```python
from build123d import *

# Parameters (mm, degrees)
F0_W           = 1549.4
F0_H           = 254
F1_DEPTH       = 12.7
F3_D           = 6.6
F3_CBORE_D     = 11.25
F3_CBORE_DEPTH = 6
F4_W           = 7.62
F4_H           = 5.5372
F6_DEPTH       = 12.7
F8_D           = 26.59126
F10_D          = 9.5758
F12_DEPTH      = 25.4
F13_R          = 9.525


with BuildPart() as f1:
    # F0 (on Front) → F1 (new body)
    with BuildSketch(Plane.XZ):
        Rectangle(F0_W, F0_H)
    extrude(amount=F1_DEPTH)

    # F3 (through all)
    with Locations(Plane.XZ.offset(12.7)):
        with Locations((-766.8006, 106.3994), (-731.8006, 106.3994), (-731.8006, 71.3994), (-766.8006, 71.3994), (-731.8006, -71.4006), (-766.8006, -71.4006), (-766.8006, -106.4006), (-731.8006, -106.4006), (731.7994, 106.3994), (766.7994, 106.3994), (766.7994, 71.3994), (731.7994, 71.3994), (731.7994, -71.4006), (766.7994, -71.4006), (766.7994, -106.4006), (731.7994, -106.4006)):
            CounterBoreHole(F3_D / 2, F3_CBORE_D / 2, F3_CBORE_DEPTH)

    # F4 (on face) + F5 (on face) → F6 (join)
    with BuildSketch(Plane.XZ.offset(12.7)):
        with Locations((-12.1412, 0)):
            Rectangle(F4_W, F4_H)
        with BuildLine():
            Line((-15.9512, -2.7686), (-15.9512, 2.7686))
            ThreePointArc((-15.9512, 2.7686), (-18.7198, 0), (-15.9512, -2.7686))
        make_face()
        with BuildLine():
            ThreePointArc((-8.3312, -2.7686), (-5.5626, 0), (-8.3312, 2.7686))
            Line((-8.3312, 2.7686), (-8.3312, -2.7686))
        make_face()
        with Locations((12.8588, 0)):
            Rectangle(F4_W, F4_H)
        with BuildLine():
            ThreePointArc((9.0488, 2.7686), (6.2802, 0), (9.0488, -2.7686))
            Line((9.0488, -2.7686), (9.0488, 2.7686))
        make_face()
        with BuildLine():
            Line((16.6688, 2.7686), (16.6688, -2.7686))
            ThreePointArc((16.6688, -2.7686), (19.4374, 0), (16.6688, 2.7686))
        make_face()
        with BuildLine():
            Line((16.6688, -60.7314), (16.6688, -66.2686))
            ThreePointArc((16.6688, -66.2686), (19.4374, -63.5), (16.6688, -60.7314))
        make_face()
        with Locations((12.8588, -63.5)):
            Rectangle(F4_W, F4_H)
        with BuildLine():
            ThreePointArc((9.0488, -60.7314), (6.2802, -63.5), (9.0488, -66.2686))
            Line((9.0488, -66.2686), (9.0488, -60.7314))
        make_face()
        with BuildLine():
            Line((-8.3312, -60.7314), (-8.3312, -66.2686))
            ThreePointArc((-8.3312, -66.2686), (-5.5626, -63.5), (-8.3312, -60.7314))
        make_face()
        with Locations((-12.1412, -63.5)):
            Rectangle(F4_W, F4_H)
        with BuildLine():
            ThreePointArc((-15.9512, -60.7314), (-18.7198, -63.5), (-15.9512, -66.2686))
            Line((-15.9512, -66.2686), (-15.9512, -60.7314))
        make_face()
    with BuildSketch(Plane.XZ.offset(12.7)):
        Polygon((685.8, -127), (-685.8, -127), (-533.4, -279.4), (533.4, -279.4), align=None)
    extrude(amount=-F6_DEPTH)

    # F8 (through all)
    with Locations(Plane.XZ.offset(12.7)):
        with Locations((-635, -76.2), (635, -76.2)):
            Hole(F8_D / 2)

    # F10 (through all)
    with Locations(Plane.XZ.offset(12.7)):
        with Locations((-609.6, -25.4), (-609.6, -177.8), (-457.2, 88.9), (457.2, 88.9), (609.6, -25.4), (609.6, -177.8), (-304.8, -25.4), (304.8, -25.4), (0, -177.8)):
            Hole(F10_D / 2)

    # F11 (on face) → F12 (cut)
    with BuildSketch(Plane.XZ.offset(12.7)):
        Polygon((-152.4, 76.2), (-304.8, 76.2), (-152.4, -76.2), align=None)
        Polygon((152.4, -76.2), (304.8, 76.2), (152.4, 76.2), align=None)
        Polygon((355.6, -76.2), (203.2, -228.6), (355.6, -228.6), align=None)
        Polygon((-203.2, -228.6), (-355.6, -76.2), (-355.6, -228.6), align=None)
    extrude(amount=-F12_DEPTH, mode=Mode.SUBTRACT)

    # F13
    f13_edges = [f1.edges().sort_by_distance(p)[0] for p in [
        (-304.8, -6.35, 76.2),
        (-152.4, -6.35, 76.2),
        (-355.6, -6.35, -76.2),
        (-152.4, -6.35, -76.2),
        (-355.6, -6.35, -228.6),
        (-203.2, -6.35, -228.6),
        (355.6, -6.35, -228.6),
        (152.4, -6.35, 76.2),
        (152.4, -6.35, -76.2),
        (203.2, -6.35, -228.6),
        (304.8, -6.35, 76.2),
        (355.6, -6.35, -76.2),
    ]]
    fillet(f13_edges, radius=F13_R)


solid = f1.part
```
Geometry check sheet. Reference: the model listing, model coordinates, mm. A direction names the side the tool comes from. Round coordinates to 2 decimals unless told otherwise and drop trailing zeros. Loops run counter-clockwise (first coordinate to the right, second up) from the corner with the lowest first, then second, coordinate; pieces in that order, holes last. Notation, with made-up numbers: M -19,32 L 2,32 A35 ccw 2,67 Z; hole C 40,34.25 d4. An arc over 180 degrees is marked long. Return JSON: item names as keys, results as strings. Group by question number.
(1) Mould release check, pull along Z, two halves, no side actions. Record for faces 1 (the face through (-11, 0, -73)), 2 (the face through (227.8, -6.4, -0.8)), 3 (the face through (-610.7, -6.4, -202.1)): pulls with the +Z half, pulls with the -Z half, needs draft (parallel to the pull), parting line crosses it, or undercut.
(2) Scan lines: line 1 along Z through (x, y) = (304.8, -4.75); line 2 along X through (y, z) = (-7, -126); line 3 along Z through (x, y) = (-639.5, -6.5). Record each from-to range of solid material in increasing order. Write a range as [from, to].
(3) Section check B-B, the plane y = -9.75. Give the number of separate pieces and of enclosed holes in the cut face, and give its area (3 significant figures).
(4) Section check A-A, the plane z = 8. Enter the section's corners in (x, y), and give its area (3 significant figures).
(5) Set-up check for faces 4 (the face through (-11, -12.7, -73)), 5 (the face through (-229.4, -6.4, 0.8)): record each of +Z, -Z, +X, -X, +Y, -Y from which the full face is reachable in a straight line by a thin tool's end or side.
(6) Go/stop test with flat-tipped pins: pin 1 (8 mm diameter, centred on x = -74.5, z = 52.5, fed in from +Y); pin 2 (9 mm diameter, centred on x = -766.5, z = 72, fed in from -Y); pin 3 (6 mm diameter, centred on x = -766.8, z = -106.4, fed in from +Y); pin 4 (6.5 mm diameter, centred on y = -8, z = -141.5, fed in from -X). Record where each tip stops, or that it passes through.
Data:
{
 "1": {"face 1": "needs draft", "face 2": "undercut", "face 3": "pulls with the -Z half"},
 "2": {"line 1": "[-279.4, -228.6], [-127, -30.19], [-20.61, 127]", "line 2": "[-774.7, -355.6], [-305.8, 305.8], [355.6, 774.7]", "line 3": "[-173.3, -88.71], [-63.69, 127]"},
 "3": {"separate pieces": "1", "enclosed holes": "31", "area": "531,000 mm²"},
 "4": {"outline": "M -774.7,-12.7 L -236.6,-12.7 L -236.6,0 L -774.7,0 Z; M -152.4,-12.7 L 152.4,-12.7 L 152.4,0 L -152.4,0 Z; M 236.6,-12.7 L 774.7,-12.7 L 774.7,0 L 236.6,0 Z", "area": "17,500 mm²"},
 "5": {"face 4": "+Z, -Z, +X, -X, -Y", "face 5": "+Y, -Y"},
 "6": {"pin 1": "y = 0", "pin 2": "y = -6.7", "pin 3": "through", "pin 4": "x = -674.55"}
}
